Geometry check sheet. Reference: drawing and pictorial views, mm from the part's lowest x, y, z. Give positions to 0.01 mm unless a question says otherwise; leave off trailing zeros. Order: outer loops, then holes, each group sorted by start corner. A loop starts at its lowest first (then second) coordinate and runs counter-clockwise, first axis right, second up. Notation, with made-up numbers: M 12.25,24 L 59.25,24 A27 cw 59.25,63 Z; hole C -11,43 d7. An arc over 180 degrees is marked long. Use CSV: the item, a comma, the result in double quotes. Start each with the question number.
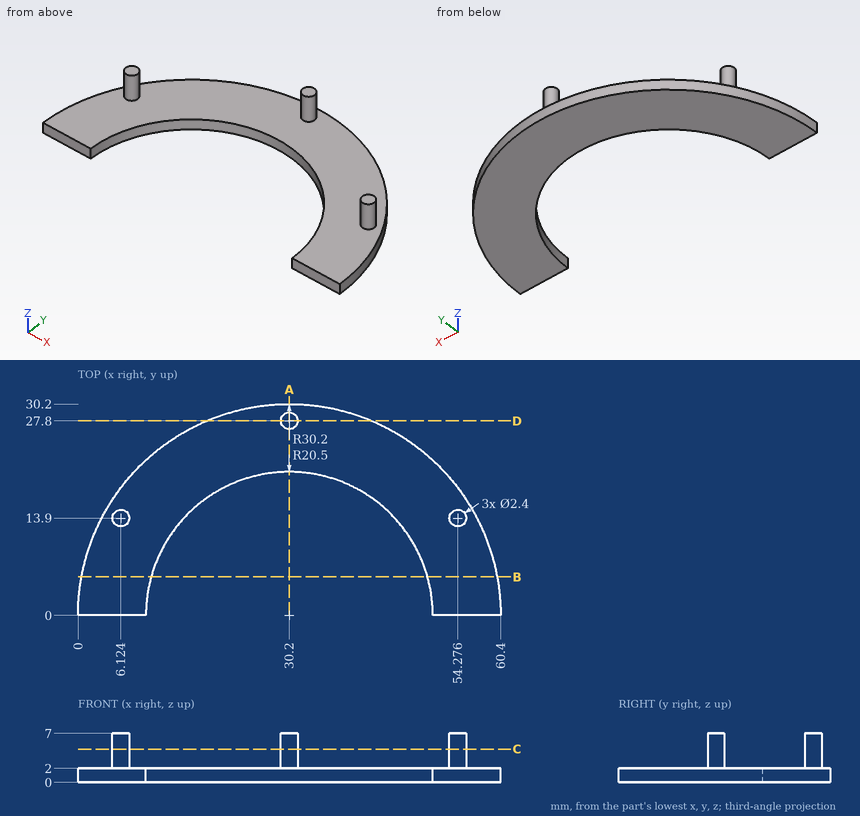
(1) Sectioned sample at A-A on x = 30.2. Record the cut outline in (y, z), then the cut area to 3 significant figures.
(2) Sectioned sample at C-C on z = 4.75. Record the cut outline in (x, y) (1 decimal).
(3) Go/stop test with flat-tipped pins: P1, Ø3, axis at y = 10.5, z = 1.5, coming from the +X side; P2, Ø2, axis at y = 21.5, z = 1.5, coming from the +X side (1 decimal). Record where each tip stops, or that it passes through.
(4) Sectioned sample at D-D on y = 27.8. Record the cut outline in (x, z).
(5) Thickness scan on line 1 (X direction, y = 14, z = 3); line 2 (Z direction, x = 27, y = 24); line 3 (X direction, y = 12.5, z = 1.5). Record the ranges inside material, lowest first.
(6) Sectioned sample at B-B on y = 5.5. Record the cut outline in (x, z) (1 decimal).
Responses:
1,outline,"M 20.5,0 L 30.2,0 L 30.2,2 L 29,2 L 29,7 L 26.6,7 L 26.6,2 L 20.5,2 Z"
1,area,"31.4 mm2"
2,outline,"C 6.1,13.9 d2.4; C 30.2,27.8 d2.4; C 54.3,13.9 d2.4"
3,P1,"x = 59.03"
3,P2,"x = 52.4"
4,outline,"M 18.4,0 L 42,0 L 42,2 L 31.4,2 L 31.4,7 L 29,7 L 29,2 L 18.4,2 Z"
5,line 1,"4.93 to 7.32, 53.08 to 55.47"
5,line 2,"0 to 2"
5,line 3,"2.71 to 13.95, 46.45 to 57.69"
6,outline,"M 0.5,0 L 10.5,0 L 10.5,2 L 0.5,2 Z; M 49.9,0 L 59.9,0 L 59.9,2 L 49.9,2 Z"
